from build123d import *

# Parameters (mm, degrees)
F0_R     = 38.131221
F1_DEPTH = 88.9
F2_R     = 25.4
F4_DEPTH = 76.2


with BuildPart() as f1:
    # F0 (on Top) → F1 (new body)
    with BuildSketch(Plane.XY):
        Circle(F0_R)
    extrude(amount=F1_DEPTH)

    # F2
    f2_edges = [f1.edges().sort_by_distance(p)[0] for p in [
        (-38.131221, 0, 88.9),
    ]]
    fillet(f2_edges, radius=F2_R)

    # F3 (on Right) → F4 (join)
    with BuildSketch(Plane.YZ):
        Polygon((4.519497, 4.251661), (5.16514, 62.359482), (-5.165141, 62.359482), (-5.165141, 4.251661), align=None)
    extrude(amount=F4_DEPTH)


solid = f1.part
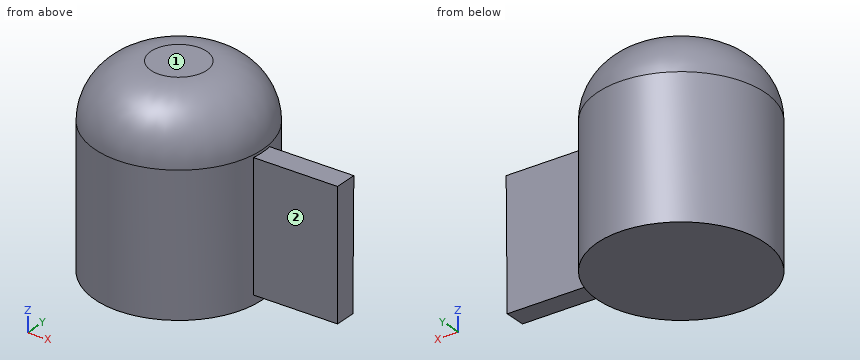
Read the model definition and answer for the solid it produces. Units are mm, in the model's axes. Face numbers are marked on the shaded views. A direction names the side the tool comes from. Coordinates: 2 decimals unless noted, no trailing zeros. Write each loop counter-clockwise with the first axis right and the second up, starting at its lowest first coordinate (ties: lowest second). Pieces come first, ordered by that corner, then holes. Notation, with made-up numbers: M 48.5,-5 L 69.5,-5 A23 cw 69.5,23 Z; hole C -33.5,-32.5 d7. An arc over 180 degrees is marked long. Use a Markdown table: item, result.
Q1. Straight lines are drawn through the part: L1, parallel to Y at x = 70.5, z = 5; L2, parallel to Y at x = 0.5, z = 25; L3, parallel to X at y = -32, z = 57. For each, find the intervals that lie inside material, in ascending order. Write a range as [from, to].
Answer block:
| item | result |
|---|---|
| L1 | y = [-5.17, 4.53] |
| L2 | y = [-38.13, 38.13] |
| L3 | x = [-20.74, 20.74] |
Q2. The part is cut by section B-B, the plane z = 26.5. Write down the section's boundary in (x, y).
Answer block:
| item | result |
|---|---|
| outline | M 37.78,-5.17 L 76.2,-5.17 L 76.2,4.77 L 37.83,4.77 A38.13 ccw long Z |
Q3. The part is cut by section A-A, the plane z = 53. Write down the section's boundary in (x, y).
Answer block:
| item | result |
|---|---|
| outline | M 37.78,-5.17 L 76.2,-5.17 L 76.2,5.06 L 37.79,5.06 A38.13 ccw long Z |
Q4. Which of the six approach directions +Z, -Z, +X, -X, +Y, -Y give full straight-line access (tool end or side, diameter ignored) to the marked faces 1 and 2?
Answer block:
| item | result |
|---|---|
| face 1 | +Z, +X, -X, +Y, -Y |
| face 2 | +Z, -Z, +X, -Y |
Q5. Each of these flat-tipped pins is pushed along its axis until it touches: pin 1 Ø3 at (x, y) = (49, -1.5) entering from +Z; pin 2 Ø8 at (y, z) = (29.5, 58) entering from -X; pin 3 Ø8 at (x, z) = (-24, 33.5) entering from +Y. Where does it stop, or does it pass through?
Answer block:
| item | result |
|---|---|
| pin 1 | stops at z = 62.36 |
| pin 2 | stops at x = -28.35 |
| pin 3 | stops at y = 32.47 |
